from build123d import *

# Parameters (mm, degrees)
SKETCH1_W            = 19.05
SKETCH1_H            = 3.175
SKETCH1_W_2          = 5.08
SKETCH1_H_2          = 44.45
BOSS_EXTRUDE1_DEPTH  = 7.62
M4_CLEARANCE_HOLE1_D = 4.5


with BuildPart() as part:
    # Sketch1 → Boss-Extrude1 (new body)
    with BuildSketch(Plane.XY):
        with Locations((-12.065, 20.6375)):
            Rectangle(SKETCH1_W, SKETCH1_H)
        Rectangle(SKETCH1_W_2, SKETCH1_H_2)
        with Locations((-12.065, -20.6375)):
            Rectangle(SKETCH1_W, SKETCH1_H)
    extrude(amount=BOSS_EXTRUDE1_DEPTH)

    # M4 Clearance Hole1 (through all)
    with Locations(Plane(origin=(0, 22.225, 0), x_dir=(1, 0, 0), z_dir=(0, 1, 0))):
        with Locations((-13.97, -3.81), (-6.35, -3.81)):
            Hole(M4_CLEARANCE_HOLE1_D / 2)


solid = part.part
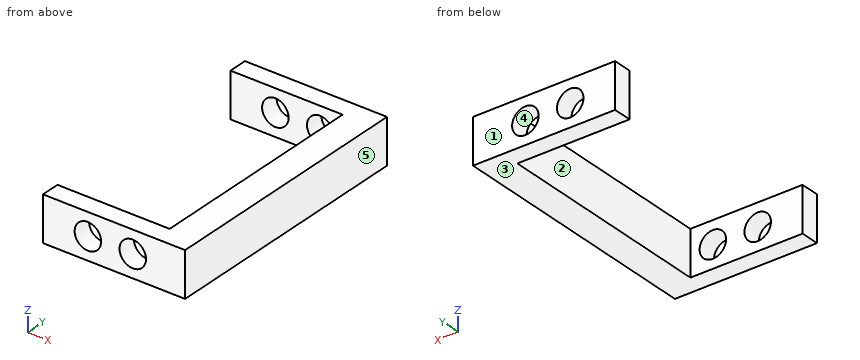
Read the model definition and answer for the solid it produces. Units are mm, in the model's axes. Face numbers are marked on the shaded views. A direction names the side the tool comes from. Give positions to 0.01 mm unless a question says otherwise; leave off trailing zeros. Write each loop counter-clockwise with the first axis right and the second up, starting at its lowest first coordinate (ties: lowest second). Pieces come first, ordered by that corner, then holes. Notation, with made-up numbers: (-12.75, 51) - (14.25, 51) arc R16 cw to (14.25, 63) - close; hole circle Ø8 at (65.25, 86). An arc over 180 degrees is marked (long way). Use CSV: the item, a comma, the result in double quotes. Start each with the question number.
(1) Find section D-D (y = 5). Give the vertices of the cut face in (x, z), plus the area to 3 significant figures.
(2) Find section C-C (x = -18.25). Give the vertices of the cut face in (y, z) (3 decimals), plus the area to 3 significant figures.
(3) Find section B-B (z = 3.81). Give the vertices of the cut face in (x, y) (3 decimals).
(4) Find section A-A (x = -6.35). Give the vertices of the cut face in (y, z) (3 decimals), plus the area to 3 significant figures.
(5) Given P1, Ø2.5, axis at x = -13.97, z = 3.81, coming from the -Y side; P2, Ø1, axis at y = 5.5, z = 6.5, coming from the -X side, each flat-ended and moving along its own axis, determine where each tip first touches the part or whether it passes through.
(6) For the marked faces 1 and 2, determine the directions among +Z, -Z, +X, -X, +Y, -Y from which every point of the face is accessible in a straight line to the end or side of a thin tool.
(7) Determine the mould class of the marked faces 3, 4 and 5 for opening direction Z: +Z half, -Z half, draft (parallel to the pull), parting line (faces both ways), or undercut.
(8) Consider line 1 along Y through (x, z) = (-17, 2) (3 decimals); line 2 along Z through (x, y) = (-13.97, -21.4); line 3 along X through (y, z) = (-8.5, 4.75). Determine where each line is inside the solid, lowest interval first.
Findings below:
1,outline,"(-2.54, 0) - (2.54, 0) - (2.54, 7.62) - (-2.54, 7.62) - close"
1,area,"38.7 mm2"
2,outline,"(-22.225, 0) - (-19.05, 0) - (-19.05, 7.62) - (-22.225, 7.62) - close; (19.05, 0) - (22.225, 0) - (22.225, 7.62) - (19.05, 7.62) - close"
2,area,"48.4 mm2"
3,outline,"(-21.59, -22.225) - (-16.22, -22.225) - (-16.22, -19.05) - (-21.59, -19.05) - close; (-21.59, 19.05) - (-16.22, 19.05) - (-16.22, 22.225) - (-21.59, 22.225) - close; (-11.72, -22.225) - (-8.6, -22.225) - (-8.6, -19.05) - (-11.72, -19.05) - close; (-11.72, 19.05) - (-8.6, 19.05) - (-8.6, 22.225) - (-11.72, 22.225) - close; (-4.1, -22.225) - (2.54, -22.225) - (2.54, 22.225) - (-4.1, 22.225) - (-4.1, 19.05) - (-2.54, 19.05) - (-2.54, -19.05) - (-4.1, -19.05) - close"
4,outline,"(-22.225, 0) - (-19.05, 0) - (-19.05, 1.56) - (-22.225, 1.56) - close; (-22.225, 6.06) - (-19.05, 6.06) - (-19.05, 7.62) - (-22.225, 7.62) - close; (19.05, 0) - (22.225, 0) - (22.225, 1.56) - (19.05, 1.56) - close; (19.05, 6.06) - (22.225, 6.06) - (22.225, 7.62) - (19.05, 7.62) - close"
4,area,"19.8 mm2"
5,P1,"through"
5,P2,"x = -2.54"
6,face 1,"+Z, -Z, +X, -X, +Y"
6,face 2,"+Z, -Z, -X"
7,face 3,"-Z half"
7,face 4,"undercut"
7,face 5,"draft"
8,line 1,"-22.225 to -19.05, 19.05 to 22.225"
8,line 2,"0 to 1.56, 6.06 to 7.62"
8,line 3,"-2.54 to 2.54"
